The model under review builds one solid part; all positions refer to its coordinate system, in mm. Give positions to 0.01 mm unless a question says otherwise; leave off trailing zeros. Order: outer loops, then holes, each group sorted by start corner. A loop starts at its lowest first (then second) coordinate and runs counter-clockwise, first axis right, second up. Notation, with made-up numbers: (17.25, 24.25) -> (43.25, 24.25) arc R12 cw to (43.25, 45.25) -> close; hole circle Ø10 at (32, 12.25). An arc over 180 degrees is marked (long way). Use one line per item in the form item = value.
```python
from build123d import *


# Not quite as in the source:
# - a feature of the source that left no trace in its solid (it failed there, or was rolled back) is left out


with BuildPart() as f2:
    # F0 (on Front) → F2 (revolve)
    with BuildSketch(Plane.XZ):
        with BuildLine():
            ThreePointArc((0.3778758058, 1.5097482936), (0.1905682406, 1.4724905024), (0, 1.46))
            ThreePointArc((0, 1.46), (-0.5587178113, 1.5711358825), (-1.0323759005, 1.8876240995))
            Line((-1.0323759005, 1.8876240995), (-22.680285707, 23.5355339059))
            ThreePointArc((-22.680285707, 23.5355339059), (-24.3024024511, 24.6193976626), (-26.2158196129, 25))
            Line((-26.2158196129, 25), (-66.445, 25))
            Line((-66.445, 25), (-66.445, 0))
            Line((-66.445, 0), (0, 0))
            Line((0, 0), (1.77, 0))
            Line((1.77, 0), (1.77, 1.8827668472))
            Line((1.77, 1.8827668472), (0.3778758058, 1.5097482936))
        make_face()
    revolve(axis=Axis((-33.2225, 0, 0), (-1, 0, 0)))


solid = f2.part
```
1. The part is to be moulded in two halves that separate along X. For faces 1 (the face through (-66.445, 0, 0)), 2 (the face through (1.77, 0, 0)), 3 (the face through (0.6, 0.471, 1.497)), say which applies: +X half, -X half, draft (parallel to the pull), parting line (faces both ways), or undercut.
Values:
face_1 = -X half
face_2 = +X half
face_3 = undercut
2. For pin 1 Ø4 at (x, z) = (-7, 8.5) entering from -Y; pin 2 Ø3 at (x, z) = (-19, -16) entering from +Y; pin 3 Ø10 at (x, z) = (-46, -15.5) entering from -Y; pin 4 Ø2 at (x, z) = (-6.5, 9.5) entering from +Y, all flat-tipped, find the tip position at first contact; note any pin that passes through.
Values:
pin_1 = -6.01
pin_2 = 14.67
pin_3 = -22.69
pin_4 = through
3. Add section A-A on x = -46. Give the boundary of the cut face in (y, z), then the cut area to 3 significant figures.
Values:
outline = circle Ø50 at (0, 0)
area = 1,960 mm^2
4. For L1, parallel to Z at x = -14.5, y = -11.5; L2, parallel to Z at x = -13, y = 3; L3, parallel to X at y = 16.5, z = -2 (3 decimals), list the stretches that pass through material, from the lowest coordinate up.
Values:
L1 = -10.18 to 10.18
L2 = -13.53 to 13.53
L3 = -66.445 to -15.766
